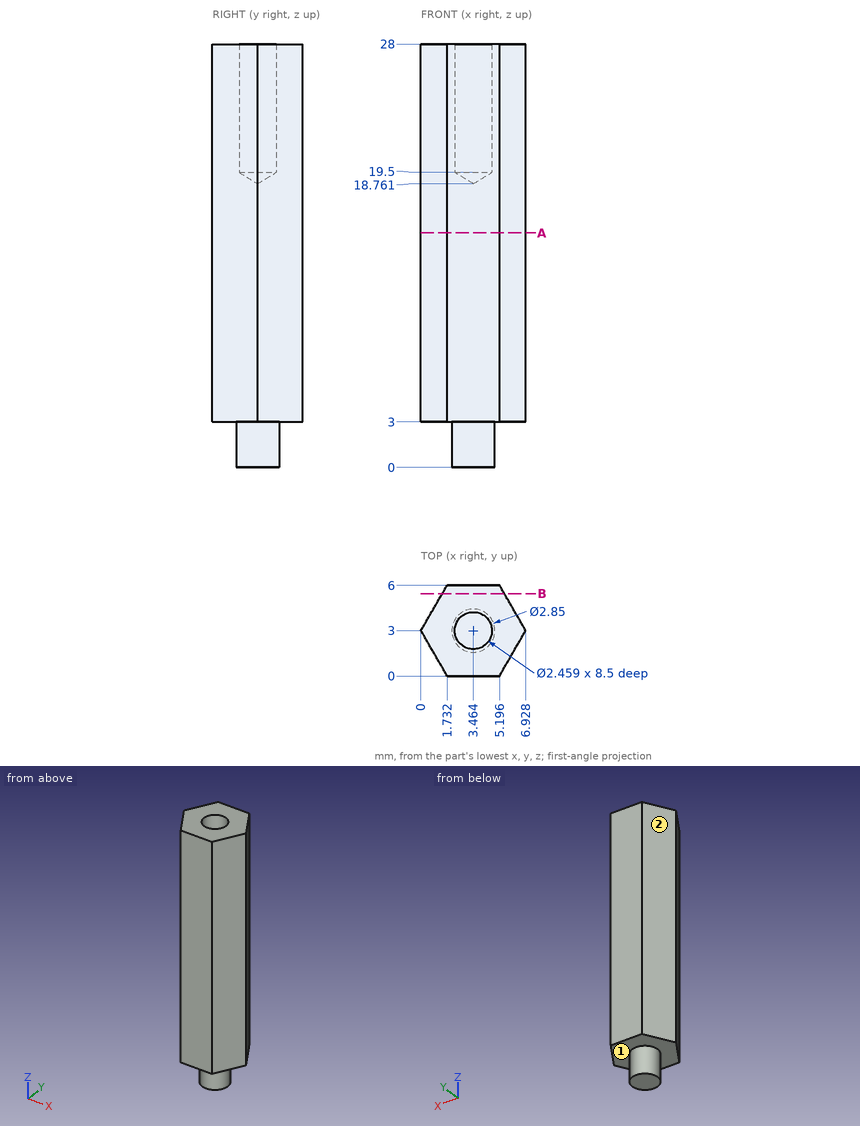
Input: dimensioned drawing with shaded views. Units: mm. Origin: part minimum x, y, z. A direction names the side the tool comes from. Give positions to 0.01 mm unless a question says otherwise; leave off trailing zeros. Loops run counter-clockwise (first coordinate to the right, second up) from the corner with the lowest first, then second, coordinate; pieces in that order, holes last. Notation, with made-up numbers: (41.5, -24.5) -> (98.5, -24.5) arc R24 cw to (98.5, -0.5) -> close; hole circle Ø2 at (68.5, 64.25). An arc over 180 degrees is marked (long way). Return JSON: item names as keys, results as strings.
Item 1: Pin query (flat end, axial travel): P1, Ø2, axis at y = 1.5, z = 10, coming from the +X side. Return the tip coordinate at first contact, or that it passes through.
Filled in:
{"P1": "x = 6.64"}
Item 2: Section B-B, the plane y = 5.45. Output: boundary loops of the cut face in (x, z).
Filled in:
{"outline": "(1.41, 3) -> (5.51, 3) -> (5.51, 28) -> (1.41, 28) -> close"}
Item 3: Line query: line 1 (Z direction, x = 1.5, y = 4.8); line 2 (X direction, y = 2.55, z = 23.75); line 3 (Y direction, x = 5.75, z = 17). Output: solid intervals per line, ascending.
Filled in:
{"line 1": "3 to 28", "line 2": "0.26 to 2.32, 4.61 to 6.67", "line 3": "0.96 to 5.04"}
Item 4: Access query for the marked faces 1 and 2. Directions: +Z, -Z, +X, -X, +Y, -Y. A direction counts if a zero-diameter tool reaches every point of the face in a straight line with its end or side. Return the directions, or none.
Filled in:
{"face 1": "-Z", "face 2": "+Z, -Z, -X, +Y"}
Item 5: Section A-A, the plane z = 15.5. Output: boundary loops of the cut face in (x, y).
Filled in:
{"outline": "(0, 3) -> (1.73, 0) -> (5.2, 0) -> (6.93, 3) -> (5.2, 6) -> (1.73, 6) -> close"}
